Verification items for the finished model (mm, model axes). A direction names the side the tool comes from. Give positions to 0.01 mm unless a question says otherwise; leave off trailing zeros. Order: outer loops, then holes, each group sorted by start corner. A loop starts at its lowest first (then second) coordinate and runs counter-clockwise, first axis right, second up.
from build123d import *

# Parameters (mm, degrees)
ESBO_O1_R                = 30
RESSALTO_EXTRUS_O1_DEPTH = 19.02
ESBO_O2_R                = 26
CORTE_EXTRUS_O1_DEPTH    = 7
ESBO_O7_R                = 27
CORTE_EXTRUS_O4_DEPTH    = 7.5
ESBO_O13_R               = 3
ESBO_O13_R_2             = 2.5
CORTE_EXTRUS_O10_DEPTH   = 12.52
ESBO_O14_R               = 4
CORTE_EXTRUS_O11_DEPTH   = 12.52
ESBO_O16_R               = 5.25
ESBO_O16_R_2             = 4.5
CORTE_EXTRUS_O12_DEPTH   = 6


with BuildPart() as part:
    # Esboço1 → Ressalto-extrusão1 (new body)
    with BuildSketch(Plane.XY):
        Circle(ESBO_O1_R)
    extrude(amount=RESSALTO_EXTRUS_O1_DEPTH)

    # Esboço2 → Corte-extrusão1 (cut)
    with BuildSketch(Plane.XY.offset(19.02)):
        Circle(ESBO_O2_R)
    extrude(amount=-CORTE_EXTRUS_O1_DEPTH, mode=Mode.SUBTRACT)

    # Esboço7 → Corte-extrusão4 (cut)
    with BuildSketch(Plane.XY.offset(19.02)):
        Circle(ESBO_O7_R)
    extrude(amount=-CORTE_EXTRUS_O4_DEPTH, mode=Mode.SUBTRACT)

    # Esboço13 → Corte-extrusão10 (cut, through all)
    with BuildSketch(Plane.XY.offset(11.52)):
        with Locations((0, 16)):
            Circle(ESBO_O13_R)
        with Locations((0, -16)):
            Circle(ESBO_O13_R)
        with Locations((-11.313708499, 11.313708499)):
            Circle(ESBO_O13_R_2)
        with Locations((11.313708499, 11.313708499)):
            Circle(ESBO_O13_R_2)
        with Locations((-11.313708499, -11.313708499)):
            Circle(ESBO_O13_R_2)
        with Locations((11.313708499, -11.313708499)):
            Circle(ESBO_O13_R_2)
    extrude(amount=-CORTE_EXTRUS_O10_DEPTH, mode=Mode.SUBTRACT)

    # Esboço14 → Corte-extrusão11 (cut, through all)
    with BuildSketch(Plane.XY.offset(11.52)):
        Circle(ESBO_O14_R)
    extrude(amount=-CORTE_EXTRUS_O11_DEPTH, mode=Mode.SUBTRACT)

    # Esboço16 → Corte-extrusão12 (cut)
    with BuildSketch(Plane(origin=(0, 0, 0), x_dir=(-1, 0, 0), z_dir=(0, 0, -1))):
        with Locations((0, 16)):
            Circle(ESBO_O16_R)
        with Locations((0, -16)):
            Circle(ESBO_O16_R)
        with Locations((11.313708499, 11.313708499)):
            Circle(ESBO_O16_R_2)
        with Locations((-11.313708499, 11.313708499)):
            Circle(ESBO_O16_R_2)
        with Locations((-11.313708499, -11.313708499)):
            Circle(ESBO_O16_R_2)
        with Locations((11.313708499, -11.313708499)):
            Circle(ESBO_O16_R_2)
    extrude(amount=-CORTE_EXTRUS_O12_DEPTH, mode=Mode.SUBTRACT)


solid = part.part
(1) Section check B-B, the plane y = -1. Enter the section's corners in (x, z).
Solved:
outline: (-29.98, 0) - (-3.87, 0) - (-3.87, 11.52) - (-26.98, 11.52) - (-26.98, 19.02) - (-29.98, 19.02) - close; (3.87, 0) - (29.98, 0) - (29.98, 19.02) - (26.98, 19.02) - (26.98, 11.52) - (3.87, 11.52) - close
(2) Go/stop test with flat-tipped pins: pin 1 (8 mm diameter, centred on y = -5.5, z = 2, fed in from +X); pin 2 (8 mm diameter, centred on x = 11.31, y = -11.31, fed in from +Z); pin 3 (5 mm diameter, centred on x = -0.5, y = 14.5, fed in from -Z). Record where each tip stops, or that it passes through.
Solved:
pin 1: stops at x = 29.96
pin 2: stops at z = 11.52
pin 3: stops at z = 6
(3) Section check C-C, the plane z = 8.5. Enter the section's corners in (x, y), then the cut area to 3 significant figures.
Solved:
outline: circle Ø60 at (0, 0); hole circle Ø5 at (-11.31, -11.31); hole circle Ø5 at (-11.31, 11.31); hole circle Ø8 at (0, 0); hole circle Ø6 at (0, -16); hole circle Ø6 at (0, 16); hole circle Ø5 at (11.31, -11.31); hole circle Ø5 at (11.31, 11.31)
area: 2,640 mm2
(4) Release check for a two-part mould opening along X. For faces 1 (the flat face through (-25, 11, 19.02)), 2 (the cylindrical face through (10.988, 13.792, 8.799)) record: pulls with the +X half, pulls with the -X half, needs draft (parallel to the pull), parting line crosses it, or undercut.
Solved:
face 1: needs draft
face 2: undercut
(5) Set-up check for faces 3 (the cylindrical face through (-13.39, 7.32, 2.96)), 4 (the cylindrical face through (13.698, -10.563, 8.799)), 5 (the cylindrical face through (-5.85, -26.36, 15.32)): record each of +Z, -Z, +X, -X, +Y, -Y from which the full face is reachable in a straight line by a thin tool's end or side.
Solved:
face 3: -Z
face 4: +Z, -Z
face 5: +Z
(6) Section check A-A, the plane x = 0. Enter the section's corners in (y, z).
Solved:
outline: (-30, 0) - (-21.25, 0) - (-21.25, 6) - (-19, 6) - (-19, 11.52) - (-27, 11.52) - (-27, 19.02) - (-30, 19.02) - close; (-13, 6) - (-10.75, 6) - (-10.75, 0) - (-4, 0) - (-4, 11.52) - (-13, 11.52) - close; (4, 0) - (10.75, 0) - (10.75, 6) - (13, 6) - (13, 11.52) - (4, 11.52) - close; (19, 6) - (21.25, 6) - (21.25, 0) - (30, 0) - (30, 19.02) - (27, 19.02) - (27, 11.52) - (19, 11.52) - close
(7) Section check D-D, the plane z = 12.75. Enter the section's corners in (x, y), then the cut area to 3 significant figures.
Solved:
outline: circle Ø60 at (0, 0); hole circle Ø54 at (0, 0)
area: 537 mm2
(8) Scan lines: line 1 (Y direction, x = 0, z = 8.25); line 2 (Y direction, x = 0, z = 4.4); line 3 (X direction, y = 8, z = 5.75). Record each from-to range of solid material in increasing order.
Solved:
line 1: y = -30 to -19, -13 to -4, 4 to 13, 19 to 30
line 2: y = -30 to -21.25, -10.75 to -4, 4 to 10.75, 21.25 to 30
line 3: x = -28.91 to -14.36, -8.27 to 8.27, 14.36 to 28.91
